Geometry check sheet. Reference: the model listing, model coordinates, mm. Face numbers are marked on the shaded views. A direction names the side the tool comes from. Round coordinates to 2 decimals unless told otherwise and drop trailing zeros. Order: outer loops, then holes, each group sorted by start corner. A loop starts at its lowest first (then second) coordinate and runs counter-clockwise, first axis right, second up.
(1) Draft check along Z on the marked faces 5, 6 and 7. Enter one of: pulls with the +Z half, pulls with the -Z half, needs draft (parallel to the pull), parting line crosses it, or undercut.
(2) Set-up check for the marked faces 1, 2, 3 and 4: record each of +Z, -Z, +X, -X, +Y, -Y from which the full face is reachable in a straight line by a thin tool's end or side.
(3) Cross-section at A-A on z = 0. Enter the section's corners in (x, y) (1 decimal), and give its area (3 significant figures).
(4) Cross-section at D-D on z = -29. Enter the section's corners in (x, y).
(5) Gauge pin test, flat ends, axial feed: P1, Ø2, axis at y = 0.5, z = -0.5, coming from the -X side; P2, Ø1, axis at y = 26, z = -17, coming from the -X side; P3, Ø22, axis at y = 20, z = -4.5, coming from the -X side (3 decimals). Record the tip position at first contact, or that the pin passes through.
(6) Cross-section at C-C on y = 47. Enter the section's corners in (x, z), and give its area (3 significant figures).
(7) Thickness scan on L1, parallel to Y at x = 17, z = -13; L2, parallel to X at y = 37.5, z = 20; L3, parallel to X at y = 11, z = 13.5 (1 decimal). Record the ranges inside material, lowest first.
from build123d import *

# Parameters (mm, degrees)
SKETCH1_W           = 17.145
SKETCH1_H           = 18.542
SKETCH2_R           = 3.71475
CUT_EXTRUDE1_DEPTH  = 8.5725
BOSS_EXTRUDE1_DEPTH = 8.5725
SKETCH4_R           = 4.45
BOSS_EXTRUDE3_DEPTH = 46


with BuildPart() as part:
    # Sketch1 → Revolve1 (revolve)
    with BuildSketch(Plane.XY):
        with Locations((16.8275, 9.271)):
            Rectangle(SKETCH1_W, SKETCH1_H)
    revolve(axis=Axis((8.255, 0, 0), (1, 0, 0)))

    # Sketch2 → Cut-Extrude1 (cut)
    with BuildSketch(Plane.ZY.offset(-8.255)):
        Circle(SKETCH2_R)
    extrude(amount=-CUT_EXTRUDE1_DEPTH, mode=Mode.SUBTRACT)

    # Sketch3 → Boss-Extrude1 (add)
    with BuildSketch(Plane(origin=(25.4, 0, 0), x_dir=(0, 0, -1), z_dir=(1, 0, 0))):
        with BuildLine():
            Line((-20.702899344, 39.448323668), (-23.827032985, 52.708168154))
            ThreePointArc((-23.827032985, 52.708168154), (-16.334994998, 63.666100226), (-6.106605949, 55.205192121))
            Line((-6.106605949, 55.205192121), (-5.453270033, 41.770518865))
            ThreePointArc((-5.453270033, 41.770518865), (0, 36.576), (5.453270033, 41.770518865))
            Line((5.453270033, 41.770518865), (6.106605949, 55.205192121))
            ThreePointArc((6.106605949, 55.205192121), (16.334994998, 63.666100226), (23.827032985, 52.708168154))
            Line((23.827032985, 52.708168154), (20.702899344, 39.448323668))
            ThreePointArc((20.702899344, 39.448323668), (20.938893682, 32.759417922), (24.542669739, 27.119386757))
            ThreePointArc((24.542669739, 27.119386757), (36.575069792, 0.260855666), (24.926987696, -26.766566093))
            ThreePointArc((24.926987696, -26.766566093), (21.721471464, -31.520323876), (20.93336456, -37.199446597))
            Line((20.93336456, -37.199446597), (22.442795242, -53.962954235))
            ThreePointArc((22.442795242, -53.962954235), (13.789101844, -63.749144471), (4.511097805, -54.552701147))
            Line((4.511097805, -54.552701147), (4.824604712, -41.518040373))
            ThreePointArc((4.824604712, -41.518040373), (0, -36.576), (-4.824604712, -41.518040373))
            Line((-4.824604712, -41.518040373), (-4.511097805, -54.552701147))
            ThreePointArc((-4.511097805, -54.552701147), (-13.789101844, -63.749144471), (-22.442795242, -53.962954235))
            Line((-22.442795242, -53.962954235), (-20.93336456, -37.199446597))
            ThreePointArc((-20.93336456, -37.199446597), (-21.721471464, -31.520323876), (-24.926987696, -26.766566093))
            ThreePointArc((-24.926987696, -26.766566093), (-36.575069792, 0.260855666), (-24.542669739, 27.119386757))
            ThreePointArc((-24.542669739, 27.119386757), (-20.938893682, 32.759417922), (-20.702899344, 39.448323668))
        make_face()
    extrude(amount=BOSS_EXTRUDE1_DEPTH)

    # Sketch4 → Boss-Extrude3 (add)
    with BuildSketch(Plane.ZY.offset(-25.4)):
        with Locations((-15.08125, 54.76875)):
            Circle(SKETCH4_R)
        with Locations((15.08125, 54.76875)):
            Circle(SKETCH4_R)
        with Locations((-13.49375, -54.76875)):
            Circle(SKETCH4_R)
        with Locations((13.49375, -54.76875)):
            Circle(SKETCH4_R)
    extrude(amount=BOSS_EXTRUDE3_DEPTH)


solid = part.part
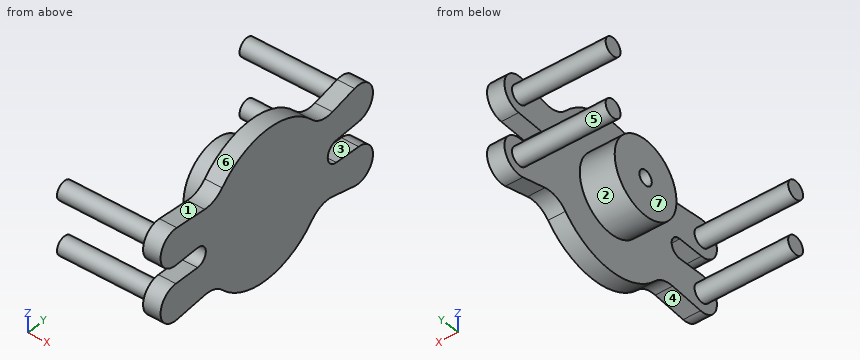
Found:
1. face 5: undercut
1. face 6: pulls with the +Z half
1. face 7: needs draft
2. face 1: +Z, +X, -X
2. face 2: -X
2. face 3: +X, -X, +Y
2. face 4: -Z, +X, -X
3. outline: (8.3, -18.5) - (25.4, -18.5) - (25.4, -36.6) - (34, -36.6) - (34, 36.6) - (25.4, 36.6) - (25.4, 18.5) - (8.3, 18.5) - (8.3, 3.7) - (16.8, 3.7) - (16.8, -3.7) - (8.3, -3.7) - close
3. area: 1,200 mm2
4. outline: (25.4, -22.29) - (33.97, -22.29) - (33.97, 22.29) - (25.4, 22.29) - close
5. P1: stops at x = 16.83
5. P2: stops at x = 25.4
5. P3: stops at x = 8.255
6. outline: (25.4, -22.48) - (33.97, -22.48) - (33.97, -5.71) - (25.4, -5.71) - close; (25.4, 5.71) - (33.97, 5.71) - (33.97, 22.48) - (25.4, 22.48) - close
6. area: 288 mm2
7. L1: y = -59.19 to -50.35, -13.22 to 13.22, 50.84 to 58.7
7. L2: x = 25.4 to 33.97
7. L3: x = 8.3 to 34
